Could you check a few things on this model? Use its own coordinates, in mm. A direction names the side the tool comes from. Give positions to 0.01 mm unless a question says otherwise; leave off trailing zeros. Write each loop counter-clockwise with the first axis right and the second up, starting at its lowest first coordinate (ties: lowest second). Pieces come first, ordered by that corner, then holes. Notation, with made-up numbers: M 50,24 L 91,24 A15 ccw 91,32 Z; hole C 77.5,58 d2. An arc over 180 degrees is marked long. Use one line per item in the form item = value.
from build123d import *

# Parameters (mm, degrees)
SKETCH1_R           = 5.5
BOSS_EXTRUDE1_DEPTH = 10


with BuildPart() as part:
    # Sketch1 → Boss-Extrude1 (new body)
    with BuildSketch(Plane.XY):
        with BuildLine():
            ThreePointArc((-9.192533317, 7.713451316), (-7.713451316, -9.192533317), (9.192533317, -7.713451316))
            Line((9.192533317, -7.713451316), (50.06797235, 41))
            Line((50.06797235, 41), (135, 41))
            Line((135, 41), (135, 65))
            Line((135, 65), (38.876588555, 65))
            Line((38.876588555, 65), (-9.192533317, 7.713451316))
        make_face()
        Circle(SKETCH1_R, mode=Mode.SUBTRACT)
        with Locations((100, 53)):
            Circle(SKETCH1_R, mode=Mode.SUBTRACT)
    extrude(amount=BOSS_EXTRUDE1_DEPTH)


solid = part.part
1) I want a section at A-A, the plane x = 100. Please give me the cut outline in (y, z), plus the area to 3 significant figures.
Checked values:
outline = M 41,0 L 47.5,0 L 47.5,10 L 41,10 Z; M 58.5,0 L 65,0 L 65,10 L 58.5,10 Z
area = 130 mm2
2) I want a section at D-D, the plane x = 70. Please give me the cut outline in (y, z), plus the area to 3 significant figures.
Checked values:
outline = M 41,0 L 65,0 L 65,10 L 41,10 Z
area = 240 mm2
3) For pin 1 Ø3 at (x, z) = (35, 5) entering from +Y; pin 2 Ø2 at (y, z) = (19, 7.5) entering from -X; pin 3 Ø6 at (y, z) = (51.5, 3.5) entering from -X; pin 4 Ø2 at (x, y) = (21, 36.5) entering from -Z, each with a flat end and sliding along its axis, tell me the tip position at first contact or that it passes through.
Checked values:
pin_1 = 62.17
pin_2 = -0.56
pin_3 = 25.03
pin_4 = 0
4) Thinking about a two-plate mould opening in X: for faces 1 (the flat face through (29.34, 16.3, 4.93)), 2 (the flat face through (15.18, 36.76, 4.93)), 3 (the cylindrical face through (-1.19, -5.37, 4.93)), which applies, released by +X, released by -X, zero draft, split by the parting line, or undercut?
Checked values:
face_1 = released by +X
face_2 = released by -X
face_3 = undercut
5) If I drill on L1, parallel to Y at x = -1, z = 5.25; L2, parallel to Y at x = 78.5, z = 9.25; L3, parallel to Y at x = 97, z = 5, over which ranges is the centre line in solid material (lowest first)?
Checked values:
L1 = -11.96 to -5.41, 5.41 to 17.48
L2 = 41 to 65
L3 = 41 to 48.39, 57.61 to 65
6) I want a section at B-B, the plane z = 7. Please give me the cut outline in (x, y), plus the area to 3 significant figures.
Checked values:
outline = M -9.19,7.71 A12 ccw 9.19,-7.71 L 50.07,41 L 135,41 L 135,65 L 38.88,65 Z; hole C 0,0 d11; hole C 100,53 d11
area = 3,870 mm2
7) For faces 4 (the flat face through (92, 41, 5)), 5 (the cylindrical face through (-7.914, -9.021, 4.93)), which set-ups out of +Z, -Z, +X, -X, +Y, -Y let a thin tool reach every point of the face, with its end or its side?
Checked values:
face_4 = +Z, -Z, +X, -Y
face_5 = +Z, -Z
8) I want a section at C-C, the plane y = 53. Please give me the cut outline in (x, z).
Checked values:
outline = M 28.81,0 L 94.5,0 L 94.5,10 L 28.81,10 Z; M 105.5,0 L 135,0 L 135,10 L 105.5,10 Z
